Read the model definition and answer for the solid it produces. Units are mm, in the model's axes. A direction names the side the tool comes from. Round coordinates to 2 decimals unless told otherwise and drop trailing zeros. Order: outer loops, then holes, each group sorted by start corner. A loop starts at its lowest first (then second) coordinate and runs counter-clockwise, first axis right, second up. Notation, with made-up numbers: (50.25, 88) - (57.25, 88) arc R12 ccw to (57.25, 93) - close; hole circle Ø5 at (81, 44). An arc over 180 degrees is marked (long way). Put each result on its own line as item: value. Start each with the question number.
Q1. Section D-D on y = -38 is taken. Give the vertices of the cut face in (x, z), then the cut area to 3 significant figures.
Q2. Section A-A on x = 44 is taken. Give the vertices of the cut face in (y, z).
Q3. Each of these flat-tipped pins is pushed along its axis until it touches: pin 1 Ø1.5 at (y, z) = (-15, 57) entering from -X; pin 2 Ø12.5 at (x, z) = (34.5, 27.5) entering from +Y; pin 3 Ø19 at (y, z) = (4.5, 52) entering from +X; pin 4 Ø3 at (x, y) = (47.5, -44) entering from -Z. Where does it stop, or does it pass through?
Q4. Which of the six approach directions +Z, -Z, +X, -X, +Y, -Y give full straight-line access (tool end or side, diameter ignored) to faces 4 (the face through (-72, -45.022, 36)), 5 (the face through (-87.302, -59.176, 36.236))?
Q5. For a pull along X with two mould halves and no side action, classify faces 1 (the face through (-71, -48.022, 36)), 2 (the face through (-90.353, -58.826, 36.236)), 3 (the face through (-0.4, -22.8, 73.5)) as pulls with the +X half, pulls with the -X half, needs draft (parallel to the pull), parting line crosses it, or undercut.
Q6. Find the intervals of material crossed by line 1 along Y through (x, z) = (-5, 61); line 2 along Y through (x, z) = (-34, 65); line 3 along X through (y, z) = (3, 59), in increasing order. Write a range as from..to.
Q7. Section B-B on y = 4 is taken. Give the vertices of the cut face in (x, z).
Q8. Section C-C on x = -64.5 is taken. Give the vertices of the cut face in (y, z), then the cut area to 3 significant figures.
from build123d import *

# Parameters (mm, degrees)
SKETCH1_W           = 20.045
SKETCH1_H           = 20.045
BOSS_EXTRUDE1_DEPTH = 73.5


with BuildPart() as part:
    # Sketch1 → Boss-Extrude1 (new body)
    with BuildSketch(Plane.XY):
        Polygon((-95.192265263, -73.0225), (95.192265263, -73.0225), (85.646810718, -45.0225), (58.839075981, -45.0225), (49.634530527, -18.0225), (15.0225, -18.0225), (15.0225, 20.0225), (-15.0225, 20.0225), (-15.0225, -18.0225), (-49.634530527, -18.0225), (-58.839075981, -45.0225), (-85.646810718, -45.0225), align=None)
        Rectangle(SKETCH1_W, SKETCH1_H, mode=Mode.SUBTRACT)
        Polygon((-20, -23.0225), (20, -23.0225), (12.5, -45.0225), (-12.5, -45.0225), align=None, mode=Mode.SUBTRACT)
        Polygon((23.169537991, -23.0225), (15.669537991, -45.0225), (55.669537991, -45.0225), (48.169537991, -23.0225), align=None, mode=Mode.SUBTRACT)
        Polygon((-55.669537991, -45.0225), (-48.169537991, -23.0225), (-23.169537991, -23.0225), (-15.669537991, -45.0225), align=None, mode=Mode.SUBTRACT)
        Polygon((55.669537991, -48.0225), (48.169537991, -70.0225), (23.169537991, -70.0225), (15.669537991, -48.0225), align=None, mode=Mode.SUBTRACT)
        Polygon((-20, -70.0225), (-12.5, -48.0225), (12.5, -48.0225), (20, -70.0225), align=None, mode=Mode.SUBTRACT)
        Polygon((-15.669537991, -48.0225), (-55.669537991, -48.0225), (-48.169537991, -70.0225), (-23.169537991, -70.0225), align=None, mode=Mode.SUBTRACT)
        Polygon((51, -70.0225), (58.5, -48.0225), (83.5, -48.0225), (91, -70.0225), align=None, mode=Mode.SUBTRACT)
        Polygon((-91, -70.0225), (-83.5, -48.0225), (-58.5, -48.0225), (-51, -70.0225), align=None, mode=Mode.SUBTRACT)
    extrude(amount=BOSS_EXTRUDE1_DEPTH)


solid = part.part
Findings:
1. outline: (-56.45, 0) - (-53.28, 0) - (-53.28, 73.5) - (-56.45, 73.5) - close; (-18.06, 0) - (-14.89, 0) - (-14.89, 73.5) - (-18.06, 73.5) - close; (14.89, 0) - (18.06, 0) - (18.06, 73.5) - (14.89, 73.5) - close; (53.28, 0) - (56.45, 0) - (56.45, 73.5) - (53.28, 73.5) - close
1. area: 932 mm2
2. outline: (-73.02, 0) - (-70.02, 0) - (-70.02, 73.5) - (-73.02, 73.5) - close; (-48.02, 0) - (-45.02, 0) - (-45.02, 73.5) - (-48.02, 73.5) - close; (-23.02, 0) - (-18.02, 0) - (-18.02, 73.5) - (-23.02, 73.5) - close
3. pin 1: x = -15.02
3. pin 2: y = -18.02
3. pin 3: x = 15.02
3. pin 4: z = 0
4. face 4: +Z, -Z, -X, +Y
4. face 5: +Z, -Z
5. face 1: undercut
5. face 2: pulls with the -X half
5. face 3: needs draft
6. line 1: -73.02..-70.02, -48.02..-45.02, -23.02..-10.02, 10.02..20.02
6. line 2: -73.02..-70.02, -48.02..-45.02, -23.02..-18.02
6. line 3: -15.02..-10.02, 10.02..15.02
7. outline: (-15.02, 0) - (-10.02, 0) - (-10.02, 73.5) - (-15.02, 73.5) - close; (10.02, 0) - (15.02, 0) - (15.02, 73.5) - (10.02, 73.5) - close
8. outline: (-73.02, 0) - (-70.02, 0) - (-70.02, 73.5) - (-73.02, 73.5) - close; (-48.02, 0) - (-45.02, 0) - (-45.02, 73.5) - (-48.02, 73.5) - close
8. area: 441 mm2
